Here's the drawing with two shaded views (mm, measured from the low corner). I have some questions. A direction names the side the tool comes from. Coordinates: 2 decimals unless noted, no trailing zeros. Loops run counter-clockwise (first coordinate to the right, second up) from the corner with the lowest first, then second, coordinate; pieces in that order, holes last. Notation, with made-up numbers: (31.5, 38.25) - (45.5, 38.25) arc R32 ccw to (45.5, 66.25) - close; hole circle Ø7 at (18, 72.5). An arc over 180 degrees is marked (long way). One line per item, written item: value. Start each with the question number.
(1) On a 3-axis mill with a long thin cutter (end or side, diameter ignored), from which of +Z, -Z, +X, -X, +Y, -Y can I reach the whole of each face in a straight line? I mean the marked faces 1, 2, 3, 4 and 5. Say none if no direction works.
(2) If we section it at B-B on y = 12: Write out the boundary of the cut face in (x, z) (1 decimal), then the cut area to 3 significant figures.
(3) If I drill on line 1 along Z through (x, y) = (31.5, 72); line 2 along X through (y, z) = (19.5, 5.5) (1 decimal); line 3 along Y through (x, z) = (12, 5.5) (1 decimal), over which ranges is the centre line in solid material (lowest first)? Write a range as from..to.
(4) If we section it at A-A on y = 35: Write out the boundary of the cut face in (x, z) (1 decimal).
(5) I'm going to push flat-ended pins straight in: P1, Ø12, axis at x = 40, y = 67, coming from the -Z side; P2, Ø7.5, axis at y = 19.5, z = 2, coming from the -X side (1 decimal); P3, Ø5, axis at x = 31, z = 27.5, coming from the +Y side (1 decimal); P4, Ø2, axis at y = 16.5, z = 2, coming from the +X side. Where does each tip first touch, or does it pass through?
(6) If we mould it in two halves opening along Y, with no side actions, what happens to the marked faces 6, 7 and 8? For each: pulls with the +Y half, pulls with the -Y half, needs draft (parallel to the pull), parting line crosses it, or undercut.
(7) If we section it at C-C on z = 23: Write out the boundary of the cut face in (x, y), then the cut area to 3 significant figures.
(8) If we section it at D-D on x = 23: Write out the boundary of the cut face in (y, z) (1 decimal).
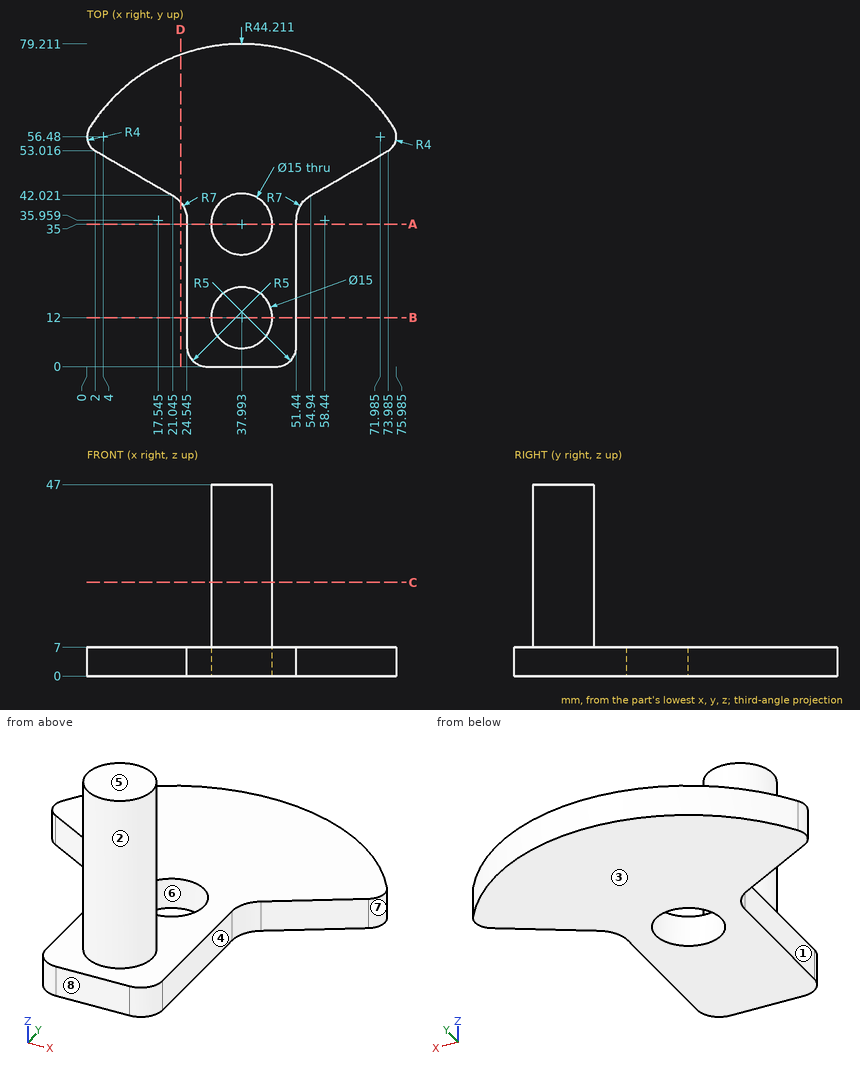
Values:
1. face 1: +Z, -Z, -X, -Y
1. face 2: +Z
1. face 3: -Z, +X, -X, +Y, -Y
1. face 4: +Z, -Z, +X, -Y
1. face 5: +Z, +X, -X, +Y, -Y
2. outline: (24.5, 0) - (51.4, 0) - (51.4, 7) - (45.5, 7) - (45.5, 47) - (30.5, 47) - (30.5, 7) - (24.5, 7) - close
2. area: 788 mm2
3. line 1: z = 0..7
3. line 2: x = 24.5..51.4
3. line 3: y = 47.2..70.8
4. outline: (24.5, 0) - (30.5, 0) - (30.5, 7) - (24.5, 7) - close; (45.5, 0) - (51.4, 0) - (51.4, 7) - (45.5, 7) - close
5. P1: stops at z = 0
5. P2: stops at x = 24.5
5. P3: stops at y = 18
5. P4: stops at x = 51.44
6. face 6: undercut
6. face 7: parting line crosses it
6. face 8: pulls with the -Y half
7. outline: circle Ø15 at (37.99, 12)
7. area: 177 mm2
8. outline: (40.3, 0) - (76.6, 0) - (76.6, 7) - (40.3, 7) - close
